from build123d import *

# Parameters (mm, degrees)
F0_W     = 76.2
F0_H     = 38.1
F1_DEPTH = 12.7
F2_W     = 12.7
F2_H     = 38.1
F3_DEPTH = 63.5
F5_D     = 15.875
F7_D     = 6.5278


with BuildPart() as f1:
    # F0 (on Top) → F1 (new body)
    with BuildSketch(Plane.XY):
        with Locations((38.1, 19.05)):
            Rectangle(F0_W, F0_H)
    extrude(amount=F1_DEPTH)

    # F2 (on face) → F3 (join)
    with BuildSketch(Plane.XY.offset(12.7)):
        with Locations((6.35, 19.05)):
            Rectangle(F2_W, F2_H)
    extrude(amount=F3_DEPTH)

    # F5 (through all)
    with Locations(Plane(origin=(0, 0, 0), x_dir=(0, -1, 0), z_dir=(-1, 0, 0))):
        with Locations((-19.05, 57.15)):
            Hole(F5_D / 2)

    # F7 (through all)
    with Locations(Plane(origin=(0, 0, 0), x_dir=(1, 0, 0), z_dir=(0, 0, -1))):
        with Locations((67.31, -19.05), (29.21, -19.05)):
            Hole(F7_D / 2)


solid = f1.part
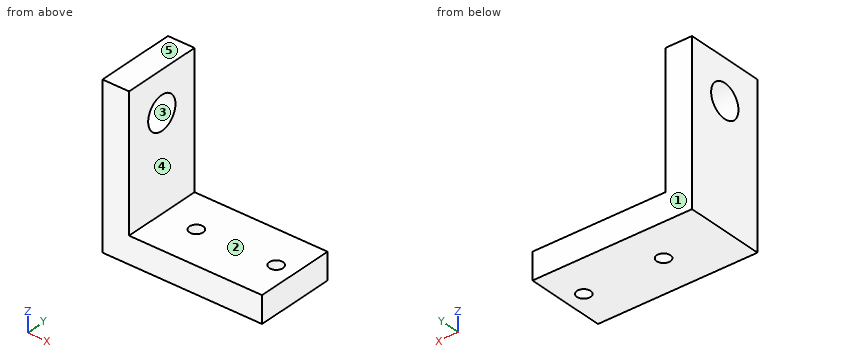
Work out the finished part from the listing and answer in its coordinate system (mm). Face numbers are marked on the shaded views. A direction names the side the tool comes from. Coordinates: 2 decimals unless noted, no trailing zeros. Loops run counter-clockwise (first coordinate to the right, second up) from the corner with the lowest first, then second, coordinate; pieces in that order, holes last. Notation, with made-up numbers: (-16.5, -22.75) -> (0.5, -22.75) arc R5 ccw to (0.5, -18.75) -> close; hole circle Ø2 at (63.5, 77.25). An arc over 180 degrees is marked (long way). Answer as CSV lines item,"result".
1) For the marked faces 4 and 5, determine the directions among +Z, -Z, +X, -X, +Y, -Y from which every point of the face is accessible in a straight line to the end or side of a thin tool.
A:
face 4,"+Z, +X, +Y, -Y"
face 5,"+Z, +X, -X, +Y, -Y"
2) The part is cut by section A-A (y = 19.05). Give the vertices of the cut face in (x, z), and give its area (3 significant figures).
A:
outline,"(0, 0) -> (25.95, 0) -> (25.95, 12.7) -> (12.7, 12.7) -> (12.7, 49.21) -> (0, 49.21) -> close; (0, 65.09) -> (12.7, 65.09) -> (12.7, 76.2) -> (0, 76.2) -> close; (32.47, 0) -> (64.05, 0) -> (64.05, 12.7) -> (32.47, 12.7) -> close; (70.57, 0) -> (76.2, 0) -> (76.2, 12.7) -> (70.57, 12.7) -> close"
area,"1,410 mm²"
3) The part is cut by section B-B (z = 57.15). Give the vertices of the cut face in (x, y), and give its area (3 significant figures).
A:
outline,"(0, 0) -> (12.7, 0) -> (12.7, 11.11) -> (0, 11.11) -> close; (0, 26.99) -> (12.7, 26.99) -> (12.7, 38.1) -> (0, 38.1) -> close"
area,"282 mm²"
4) The part is cut by section C-C (x = 67.31). Give the vertices of the cut face in (y, z), and give its area (3 significant figures).
A:
outline,"(0, 0) -> (15.79, 0) -> (15.79, 12.7) -> (0, 12.7) -> close; (22.31, 0) -> (38.1, 0) -> (38.1, 12.7) -> (22.31, 12.7) -> close"
area,"401 mm²"
5) Flat-ended cylindrical pins translate along their axes: pin 1 (4 mm diameter, centred on x = 67.31, y = 19.05, fed in from +Z); pin 2 (4 mm diameter, centred on y = 33.5, z = 64.5, fed in from +X). Find the tip coordinate at first contact, or state that the pin passes through.
A:
pin 1,"passes through"
pin 2,"stops at x = 12.7"
6) Straight lines are drawn through the part: probe 1 along X at (y, z) = (19, 7); probe 2 along X at (y, z) = (21, 3.5); probe 3 along Y at (x, z) = (29.21, 7). For each, find the intervals that lie inside material, in ascending order.
A:
probe 1,"x = 0 to 25.95, 32.47 to 64.05, 70.57 to 76.2"
probe 2,"x = 0 to 26.59, 31.83 to 64.69, 69.93 to 76.2"
probe 3,"y = 0 to 15.79, 22.31 to 38.1"
7) For a pull along Z with two mould halves and no side action, classify the marked faces 1, 2 and 3 as released by +Z, released by -Z, zero draft, split by the parting line, or undercut.
A:
face 1,"zero draft"
face 2,"released by +Z"
face 3,"undercut"
